from build123d import *

# Parameters (mm, degrees)
SKETCH1_W                = 65
SKETCH1_H                = 25
BOSS_EXTRUDE1_DEPTH      = 10
BOSS_EXTRUDE2_DEPTH      = 2.5
BOSS_EXTRUDE2_DEPTH_BACK = 67.5
SKETCH2_R                = 2


with BuildPart() as part:
    # Sketch1 → Boss-Extrude1 (new body)
    with BuildSketch(Plane(origin=(0, 0, 0), x_dir=(1, 0, 0), z_dir=(0, 1, 0))):
        Rectangle(SKETCH1_W, SKETCH1_H)
    extrude(amount=BOSS_EXTRUDE1_DEPTH)

    # Sketch2 → Boss-Extrude2 (add, two sides: drawn at the far end of the back side and taken through both)
    with BuildSketch(Plane(origin=(32.5, 0, 0), x_dir=(0, 0, -1), z_dir=(1, 0, 0)).offset(-BOSS_EXTRUDE2_DEPTH_BACK)):
        with Locations((-8.319077052, 5)):
            Circle(SKETCH2_R)
        with Locations((8.319077052, 5)):
            Circle(SKETCH2_R)
    extrude(amount=BOSS_EXTRUDE2_DEPTH + BOSS_EXTRUDE2_DEPTH_BACK)


solid = part.part
The listing builds one solid part. Answer for the finished solid, in the listing's coordinates (mm). A direction names the side the tool comes from. Give positions to 0.01 mm unless a question says otherwise; leave off trailing zeros. Loops run counter-clockwise (first coordinate to the right, second up) from the corner with the lowest first, then second, coordinate; pieces in that order, holes last.
Item 1: A cutting plane is placed at A-A (y = 5). Give the vertices of the cut face in (x, z).
Derived:
outline: (-35, -10.32) - (-32.5, -10.32) - (-32.5, -12.5) - (32.5, -12.5) - (32.5, -10.32) - (35, -10.32) - (35, -6.32) - (32.5, -6.32) - (32.5, 6.32) - (35, 6.32) - (35, 10.32) - (32.5, 10.32) - (32.5, 12.5) - (-32.5, 12.5) - (-32.5, 10.32) - (-35, 10.32) - (-35, 6.32) - (-32.5, 6.32) - (-32.5, -6.32) - (-35, -6.32) - close
Item 2: This flat-tipped pin is pushed along its axis until it touches: pin 1 Ø1 at (y, z) = (6, 3.5) entering from +X. Where does it stop, or does it pass through?
Derived:
pin 1: stops at x = 32.5
Item 3: A tool of negligible diameter and unlimited length cuts with its end or side. For faces 5 (the cylindrical face through (-33.77, 5.09, -6.32)), 6 (the cylindrical face through (33.73, 5.09, -6.32)), 7 (the flat face through (0, 10, 0)), from which of +Z, -Z, +X, -X, +Y, -Y can it reach the whole face along a straight path? Write none if from no direction.
Derived:
face 5: -X
face 6: +X
face 7: +Z, -Z, +X, -X, +Y
Item 4: Determine the mould class of faces 1 (the cylindrical face through (-33.77, 5.6, 6.41)), 2 (the flat face through (0, 5, -12.5)), 3 (the flat face through (32.5, 5, 0)), 4 (the flat face through (35, 5, 8)) for opening direction Z: +Z half, -Z half, draft (parallel to the pull), parting line (faces both ways), or undercut.
Derived:
face 1: undercut
face 2: -Z half
face 3: undercut
face 4: draft
Item 5: A cutting plane is placed at C-C (z = 8). Give the vertices of the cut face in (x, y), then the cut area to 3 significant figures.
Derived:
outline: (-35, 3.03) - (-32.5, 3.03) - (-32.5, 0) - (32.5, 0) - (32.5, 3.03) - (35, 3.03) - (35, 6.97) - (32.5, 6.97) - (32.5, 10) - (-32.5, 10) - (-32.5, 6.97) - (-35, 6.97) - close
area: 670 mm2
Item 6: Find the intervals of material crossed by line 1 along X through (y, z) = (0.5, -6.5), in increasing order.
Derived:
line 1: x = -32.5 to 32.5
Item 7: A cutting plane is placed at D-D (y = 1.25). Give the vertices of the cut face in (x, z).
Derived:
outline: (-32.5, -12.5) - (32.5, -12.5) - (32.5, 12.5) - (-32.5, 12.5) - close
Item 8: A cutting plane is placed at B-B (z = -0.75). Give the vertices of the cut face in (x, y).
Derived:
outline: (-32.5, 0) - (32.5, 0) - (32.5, 10) - (-32.5, 10) - close
